Build history of the part. All positions in model axes, mm. Face numbers are marked on the shaded views. A direction names the side the tool comes from. Round coordinates to 2 decimals unless told otherwise and drop trailing zeros. Write each loop counter-clockwise with the first axis right and the second up, starting at its lowest first coordinate (ties: lowest second). Pieces come first, ordered by that corner, then holes.
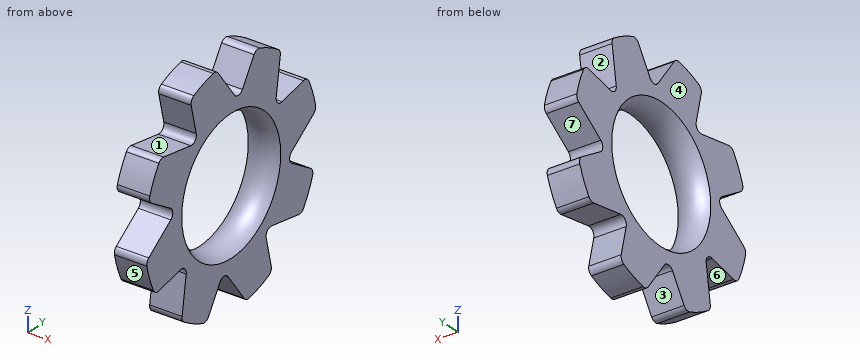
from build123d import *

# Parameters (mm, degrees)
F4_DEPTH = 60
F5_R     = 5


# Not quite as in the source:
# - a feature names something its author has since deleted; it is built from what else it names


with BuildPart() as f1:
    # F0 (on Top) → F1 (revolve)
    with BuildSketch(Plane.XY):
        with BuildLine():
            Line((-12.5, 89.1), (-12.5, 51.1))
            ThreePointArc((-12.5, 51.1), (0, 46.135443521), (12.5, 51.1))
            Line((12.5, 51.1), (12.5, 89.1))
            Line((12.5, 89.1), (-12.5, 89.1))
        make_face()
    revolve(axis=Axis((4.8881422824, 0, 0), (1, 0, 0)))

    # F3 (on offset) → F4 (cut)
    with BuildSketch(Plane.YZ.offset(15)):
        Polygon((43.1796096184, -82.538823422), (80.155778704, -52.2855824361), (34.4793311693, -45.3649125185), align=None)
        Polygon((-27.8311669827, -88.896356523), (19.707204774, -93.6501845717), (-7.6972683892, -56.4584061503), align=None)
        Polygon((-82.538823422, -43.1796096184), (-52.2855824361, -80.155778704), (-45.3649125185, -34.4793311693), align=None)
        Polygon((-56.4584061503, 7.6972683892), (-88.896356523, 27.8311669827), (-93.6501845717, -19.707204774), align=None)
        Polygon((-43.1796096184, 82.538823422), (-80.155778704, 52.2855824361), (-34.4793311693, 45.3649125185), align=None)
        Polygon((27.8311669827, 88.896356523), (-19.707204774, 93.6501845717), (7.6972683892, 56.4584061503), align=None)
        Polygon((82.538823422, 43.1796096184), (52.2855824361, 80.155778704), (45.3649125185, 34.4793311693), align=None)
        Polygon((88.896356523, -27.8311669827), (93.6501845717, 19.707204774), (56.4584061503, -7.6972683892), align=None)
    extrude(amount=-F4_DEPTH, mode=Mode.SUBTRACT)

    # F5
    f5_edges = [f1.edges().sort_by_distance(p)[0] for p in [
        (0, 87.764267, 15.370212),
        (0, 85.336625, -25.621679),
        (0, 72.92709, -51.190327),
        (0, 78.459369, 42.224844),
        (0, 51.190327, 72.92709),
        (0, 42.224844, -78.459369),
        (0, 15.370212, -87.764267),
        (0, 34.479331, -45.364913),
        (0, 56.458406, -7.697268),
        (0, 45.364913, 34.479331),
        (0, 25.621679, 85.336625),
        (0, 7.697268, 56.458406),
        (0, -15.370212, 87.764267),
        (0, -42.224844, 78.459369),
        (0, -34.479331, 45.364913),
        (0, -72.92709, 51.190327),
        (0, -85.336625, 25.621679),
        (0, -56.458406, 7.697268),
        (0, -87.764267, -15.370212),
        (0, -78.459369, -42.224844),
        (0, -45.364913, -34.479331),
        (0, -51.190327, -72.92709),
        (0, -25.621679, -85.336625),
        (0, -7.697268, -56.458406),
    ]]
    fillet(f5_edges, radius=F5_R)


solid = f1.part
1) Slice it at A-A (y = 72.5). Write the cut outline in (x, z), plus the area to 3 significant figures.
Results:
outline: (-12.5, -50.38) - (12.5, -50.38) - (12.5, -17.65) - (-12.5, -17.65) - close; (-12.5, 4.12) - (12.5, 4.12) - (12.5, 40.83) - (-12.5, 40.83) - close
area: 1,740 mm2
2) Wall check: L1, parallel to Y at x = -8.5, z = -33; L2, parallel to Z at x = -1.5, y = 75; L3, parallel to Y at x = -11, z = -10. Give the ranges that are in metal, low to high.
Results:
L1: y = -82.76 to -35.19, 35.19 to 82.76
L2: z = -48.1 to -19.21, 5.96 to 41.4
L3: y = -80.48 to -48.82, 48.82 to 61.13
3) Slice it at B-B (z = -77). Write the cut outline in (x, y), plus the area to 3 significant figures.
Results:
outline: (-12.5, -44.83) - (12.5, -44.83) - (12.5, -20.45) - (-12.5, -20.45) - close; (-12.5, 7.44) - (12.5, 7.44) - (12.5, 41.31) - (-12.5, 41.31) - close
area: 1,460 mm2
4) Which spindle directions (+Z, -Z, +X, -X, +Y, -Y) get a long thin tool onto all of the face, cutting with end or side? Do the marked faces 1, 2 and 3. Say none if no direction does.
Results:
face 1: +Z, +X, -X
face 2: +X, -X, +Y
face 3: -Z, +X, -X
5) Pin check, flat tips, straight feed: pin 1 Ø5 at (x, z) = (-5.5, -7.5) entering from +Y; pin 2 Ø4 at (x, y) = (3, -14.5) entering from -Z; pin 3 Ø12 at (x, y) = (8, 64) entering from +Z (3 decimals). Stop position of each tip, or through.
Results:
pin 1: stops at y = 61.13
pin 2: stops at z = -70.64
pin 3: stops at z = 40.245
6) Mould opens along Y. For the marked faces 4, 5, 6 and 7 say: released by +Y, released by -Y, zero draft, split by the parting line, or undercut.
Results:
face 4: zero draft
face 5: released by -Y
face 6: undercut
face 7: released by +Y
